```python
from build123d import *

# Parameters (mm, degrees)
F0_W     = 101.118554
F0_H     = 15
F0_R     = 3.514012
F0_R_2   = 3.175
F1_DEPTH = 25.4


with BuildPart() as f1:
    # F0 (on Front) → F1 (new body)
    with BuildSketch(Plane.XZ):
        with Locations((-2.165472, 0.328236)):
            Rectangle(F0_W, F0_H)
        with Locations((-31.025723, 0)):
            Circle(F0_R, mode=Mode.SUBTRACT)
        Circle(F0_R_2, mode=Mode.SUBTRACT)
        with Locations((27.468633, 0)):
            Circle(F0_R_2, mode=Mode.SUBTRACT)
        with BuildLine():
            Line((-52.724749, -7.171764), (-52.724749, 7.828236))
            ThreePointArc((-52.724749, 7.828236), (-58.651611, 0.328236), (-52.724749, -7.171764))
        make_face()
        with BuildLine():
            ThreePointArc((48.393805, -7.171764), (53.540338, 0.328236), (48.393805, 7.828236))
            Line((48.393805, 7.828236), (48.393805, -7.171764))
        make_face()
    extrude(amount=F1_DEPTH)


solid = f1.part
```
Part model, mm, in its own coordinate system. Round coordinates to 2 decimals unless told otherwise and drop trailing zeros. Order: outer loops, then holes, each group sorted by start corner. A loop starts at its lowest first (then second) coordinate and runs counter-clockwise, first axis right, second up. Notation, with made-up numbers: M 77,84.5 L 121,84.5 A25 cw 121,104.5 Z; hole C 2,-32.5 d1. An arc over 180 degrees is marked long. Answer in a Markdown table with one row per item. Add a question column.
Q1. Cut at D-D on x = -29.5. Give the cut face in (y, z).
Q2. Mould opens along Z. For faces 1 (the face through (-34.536, -12.522, 0.155)), 2 (the face through (-58.65, -12.52, 0.47)), 3 (the face through (-3.34, 0, 0.43)), 4 (the face through (-3, -13, 7.828)) say: +Z half, -Z half, draft (parallel to the pull), parting line (faces both ways), or undercut.
Q3. Pin check, flat tips, straight feed: pin 1 (5.5 mm diameter, centred on x = 27.47, z = 0, fed in from -Y); pin 2 (5 mm diameter, centred on y = -7, z = -4.5, fed in from +X); pin 3 (1 mm diameter, centred on y = -6.5, z = 2.5, fed in from -X); pin 4 (6 mm diameter, centred on y = -4.5, z = -5.5, fed in from -X). Stop position of each tip, or through.
Q4. Cut at A-A on x = 0. Give the cut face in (y, z) (3 decimals), and give its area (3 significant figures).
Q5. Cut at B-B on y = -11. Give the cut face in (x, z) (3 decimals), and give its area (3 significant figures).
Q6. Wall check: L1, parallel to X at y = -13, z = -0.25; L2, parallel to Z at x = 0, y = -20.5 (3 decimals); L3, parallel to Z at x = 27, y = -7.5. Give the ranges that are in metal, low to high. Write a range as from..to.
Q7. Cut at C-C on z = 0. Give the cut face in (x, y) (3 decimals), and give its area (3 significant figures).
Established:
| question | item | result |
|---|---|---|
| 1 | outline | M -25.4,-7.17 L 0,-7.17 L 0,-3.17 L -25.4,-3.17 Z; M -25.4,3.17 L 0,3.17 L 0,7.83 L -25.4,7.83 Z |
| 2 | face 1 | undercut |
| 2 | face 2 | parting line |
| 2 | face 3 | draft |
| 2 | face 4 | +Z half |
| 3 | pin 1 | passes through |
| 3 | pin 2 | stops at x = 53.2 |
| 3 | pin 3 | stops at x = -58.47 |
| 3 | pin 4 | stops at x = -58.11 |
| 4 | outline | M -25.4,-7.172 L 0,-7.172 L 0,-3.175 L -25.4,-3.175 Z; M -25.4,3.175 L 0,3.175 L 0,7.828 L -25.4,7.828 Z |
| 4 | area | 220 mm2 |
| 5 | outline | M -52.725,-7.172 L 48.394,-7.172 A8.038 ccw 48.394,7.828 L -52.725,7.828 A7.709 ccw Z; hole C -31.026,0 d7.028; hole C 0,0 d6.35; hole C 27.469,0 d6.35 |
| 5 | area | 1,540 mm2 |
| 6 | L1 | x = -58.63..-34.53, -27.52..-3.17, 3.17..24.3, 30.63..53.52 |
| 6 | L2 | z = -7.172..-3.175, 3.175..7.828 |
| 6 | L3 | z = -7.17..-3.14, 3.14..7.83 |
| 7 | outline | M -58.645,-25.4 L -34.54,-25.4 L -34.54,0 L -58.645,0 Z; M -27.512,-25.4 L -3.175,-25.4 L -3.175,0 L -27.512,0 Z; M 3.175,-25.4 L 24.294,-25.4 L 24.294,0 L 3.175,0 Z; M 30.644,-25.4 L 53.534,-25.4 L 53.534,0 L 30.644,0 Z |
| 7 | area | 2,350 mm2 |
